Build history of the part. All positions in model axes, mm. Coordinates: 2 decimals unless noted, no trailing zeros. Write each loop counter-clockwise with the first axis right and the second up, starting at its lowest first coordinate (ties: lowest second). Pieces come first, ordered by that corner, then holes.
```python
from build123d import *

# Parameters (mm, degrees)
F0_R     = 15
F1_DEPTH = 20
F2_R     = 5.08
F3_R     = 5.08
F5_D     = 12.7


with BuildPart() as f1:
    # F0 (on Front) → F1 (new body)
    with BuildSketch(Plane.XZ):
        Circle(F0_R)
    extrude(amount=F1_DEPTH)

    # F2
    f2_edges = [f1.edges().sort_by_distance(p)[0] for p in [
        (-15, -20, 0),
    ]]
    fillet(f2_edges, radius=F2_R)

    # F3
    f3_edges = [f1.edges().sort_by_distance(p)[0] for p in [
        (15, -7.46, 0),
        (-15, -14.92, 0),
        (-15, 0, 0),
    ]]
    fillet(f3_edges, radius=F3_R)

    # F5 (through all)
    with Locations(Plane(origin=(0, 0, 0), x_dir=(1, 0, 0), z_dir=(0, 1, 0))):
        with Locations((0, 0)):
            Hole(F5_D / 2)


solid = f1.part
```
1. Flat gauge pins, fed straight in: pin 1 (8 mm diameter, centred on y = -12.5, z = 9, fed in from -X); pin 2 (8 mm diameter, centred on x = 3, y = -4.5, fed in from +Z); pin 3 (12 mm diameter, centred on y = -6, z = -10.5, fed in from +X); pin 4 (8 mm diameter, centred on y = -3.5, z = -10, fed in from +X). Where does each tip first touch, or does it go through?
Computed values:
pin 1: stops at x = -14.14
pin 2: stops at z = 15
pin 3: stops at x = 14.31
pin 4: stops at x = 13.66
2. Saw through at A-A on x = 0. List the corners of the cut face in (y, z), plus the area to 3 significant figures.
Computed values:
outline: (-20, -9.92) arc R5.08 ccw to (-14.92, -15) - (-5.08, -15) arc R5.08 ccw to (0, -9.92) - (0, -6.35) - (-20, -6.35) - close; (-20, 6.35) - (0, 6.35) - (0, 9.92) arc R5.08 ccw to (-5.08, 15) - (-14.92, 15) arc R5.08 ccw to (-20, 9.92) - close
area: 324 mm2
3. Saw through at C-C on y = -6.25. List the corners of the cut face in (x, z), plus the area to 3 significant figures.
Computed values:
outline: circle Ø30 at (0, 0); hole circle Ø12.7 at (0, 0)
area: 580 mm2
4. Saw through at B-B on z = 0. List the corners of the cut face in (x, y).
Computed values:
outline: (-15, -14.92) arc R5.08 ccw to (-9.92, -20) - (-6.35, -20) - (-6.35, 0) - (-9.92, 0) arc R5.08 ccw to (-15, -5.08) - close; (6.35, -20) - (9.92, -20) arc R5.08 ccw to (15, -14.92) - (15, -5.08) arc R5.08 ccw to (9.92, 0) - (6.35, 0) - close
5. Saw through at D-D on y = -15.5. List the corners of the cut face in (x, z), plus the area to 3 significant figures.
Computed values:
outline: circle Ø29.93 at (0, 0); hole circle Ø12.7 at (0, 0)
area: 577 mm2
6. Mould opens along X. For faces 1 (the face through (-14.985, -9.931, 0.66)), 2 (the face through (1.38, -10.14, 6.2)), 3 (the face through (-0.1, 0, -6.5)) say: +X half, -X half, draft (parallel to the pull), parting line (faces both ways), or undercut.
Computed values:
face 1: parting line
face 2: undercut
face 3: draft
7. Probe line 1 along Z through (x, y) = (0, -12.5); line 2 along Z through (x, y) = (-5, -10.75); line 3 along X through (y, z) = (-8.75, 1). List the from-to ranges inside material, lowest first.
Computed values:
line 1: z = -15 to -6.35, 6.35 to 15
line 2: z = -14.14 to -3.91, 3.91 to 14.14
line 3: x = -14.97 to -6.27, 6.27 to 14.97
